from build123d import *

# Parameters (mm, degrees)
SKETCH1_W           = 381
SKETCH1_H           = 127
BOSS_EXTRUDE1_DEPTH = 25.4
FILLET1_R           = 63.5
FILLET2_R           = 38.1
BOSS_EXTRUDE2_DEPTH = 25.4
BOSS_EXTRUDE3_DEPTH = 12.7
SKETCH11_R          = 34.925
CUT_EXTRUDE4_DEPTH  = 38.1


with BuildPart() as part:
    # Sketch1 → Boss-Extrude1 (new body)
    with BuildSketch(Plane(origin=(0, 0, 0), x_dir=(1, 0, 0), z_dir=(0, 1, 0))):
        with Locations((-190.5, -63.5)):
            Rectangle(SKETCH1_W, SKETCH1_H)
    extrude(amount=BOSS_EXTRUDE1_DEPTH)

    # Fillet1
    fillet1_edges = [part.edges().sort_by_distance(p)[0] for p in [
        (0, 12.7, 0),
        (0, 12.7, 127),
    ]]
    fillet(fillet1_edges, radius=FILLET1_R - 0.0001)  # a hair under: the kernel refuses the full size

    # Fillet2
    fillet2_edges = [part.edges().sort_by_distance(p)[0] for p in [
        (-381, 12.7, 127),
        (-381, 12.7, 0),
    ]]
    fillet(fillet2_edges, radius=FILLET2_R)

    # Sketch2 → Boss-Extrude2 (add)
    with BuildSketch(Plane(origin=(0, 0, 0), x_dir=(1, 0, 0), z_dir=(0, 1, 0))):
        with BuildLine():
            Line((-63.5, -12.7), (-342.9, -11.159231637))
            Line((-342.9, -11.159231637), (-342.9, 0))
            Line((-342.9, 0), (-63.5, 0))
            ThreePointArc((-63.5, 0), (0, -63.5), (-63.5, -127))
            Line((-63.5, -127), (-342.9, -127))
            Line((-342.9, -127), (-342.9, -114.3))
            Line((-342.9, -114.3), (-63.5, -114.3))
            ThreePointArc((-63.5, -114.3), (-12.7, -63.5), (-63.5, -12.7))
        make_face()
    extrude(amount=-BOSS_EXTRUDE2_DEPTH)

    # Sketch3 → Boss-Extrude3 (add)
    with BuildSketch(Plane(origin=(0, -25.4, 0), x_dir=(1, 0, 0), z_dir=(0, 1, 0))):
        with BuildLine():
            Line((-342.9, -127), (-342.9, -82.55))
            Line((-342.9, -82.55), (-63.5, -82.55))
            ThreePointArc((-63.5, -82.55), (-44.45, -63.5), (-63.5, -44.45))
            Line((-63.5, -44.45), (-342.9, -44.45))
            Line((-342.9, -44.45), (-342.9, 0))
            Line((-342.9, 0), (-63.5, 0))
            ThreePointArc((-63.5, 0), (0, -63.5), (-63.5, -127))
            Line((-63.5, -127), (-342.9, -127))
        make_face()
    extrude(amount=-BOSS_EXTRUDE3_DEPTH)

    # Sketch11 → Cut-Extrude4 (cut)
    with BuildSketch(Plane(origin=(0, 25.4, 0), x_dir=(1, 0, 0), z_dir=(0, 1, 0))):
        with Locations(Location((-317.5, -63.5, 0), (0, 0, 270))):
            Circle(SKETCH11_R)
    extrude(amount=-CUT_EXTRUDE4_DEPTH, mode=Mode.SUBTRACT)


solid = part.part
Can you work these out from the model? Positions are in its coordinate system, mm. A direction names the side the tool comes from. Give positions to 0.01 mm unless a question says otherwise; leave off trailing zeros. Loops run counter-clockwise (first coordinate to the right, second up) from the corner with the lowest first, then second, coordinate; pieces in that order, holes last. Notation, with made-up numbers: (25, -18.75) - (74, -18.75) arc R12 ccw to (74, 2.25) - close; hole circle Ø1 at (-6, -25). An arc over 180 degrees is marked (long way). Answer as a JSON object with one key per item and string values.
Q1. Will these pins go through, and if not, where does the flat tip stop? P1, Ø4, axis at y = -4, z = 15, coming from the +X side; P2, Ø10, axis at y = -24, z = 18.5, coming from the +X side; P3, Ø11.5, axis at y = -28, z = 109.5, coming from the -X side.
Geometry says:
{"P1": "x = -20.26", "P2": "x = -14.18", "P3": "x = -342.9"}
Q2. Imagine slicing it at D-D on y = -5. Write out the boundary of the cut face in (x, z).
Geometry says:
{"outline": "(-342.9, 0) - (-63.5, 0) arc R63.5 ccw to (-63.5, 127) - (-342.9, 127) - (-342.9, 114.3) - (-63.5, 114.3) arc R50.8 cw to (-63.5, 12.7) - (-342.9, 11.16) - close"}
Q3. If we mould it in two halves opening along Z, with no side actions, what happens to faces 5 (the cylindrical face through (-19.095, 12.878, 108.892)), 6 (the flat face through (-169, -38.1, 91)), 7 (the flat face through (-201, -32, 44.45))? For each: pulls with the +Z half, pulls with the -Z half, needs draft (parallel to the pull), parting line crosses it, or undercut.
Geometry says:
{"face 5": "pulls with the +Z half", "face 6": "needs draft", "face 7": "undercut"}
Q4. Imagine slicing it at C-C on x = -349. Write out the boundary of the cut face in (y, z).
Geometry says:
{"outline": "(0, 0.49) - (25.4, 0.49) - (25.4, 48.42) - (0, 48.42) - close; (0, 78.58) - (25.4, 78.58) - (25.4, 126.51) - (0, 126.51) - close"}
Q5. Which directions (+Z, -Z, +X, -X, +Y, -Y) give clear straight access to the entire face, cutting with the end or side of a thin tool? Please do faces 1 (the cylindrical face through (-348.484, 12.878, 79.616)), 2 (the flat face through (-342.9, -27, 18)), 3 (the flat face through (-205, -13, 114.3)), 4 (the cylindrical face through (-44.455, -31.661, 63.919)).
Geometry says:
{"face 1": "+Y", "face 2": "+Z, -Z, -X, -Y", "face 3": "-X", "face 4": "-X, -Y"}
Q6. If I drill on L1, parallel to Y at x = -327, z = 110; L2, parallel to X at y = 10.25, z = 63.5 (3 decimals); L3, parallel to Z at x = -279.5, y = -30, over which ranges is the centre line in solid material (lowest first)?
Geometry says:
{"L1": "-38.1 to -25.4, 0 to 25.4", "L2": "-381 to -352.425, -282.575 to 0", "L3": "0 to 44.45, 82.55 to 127"}
